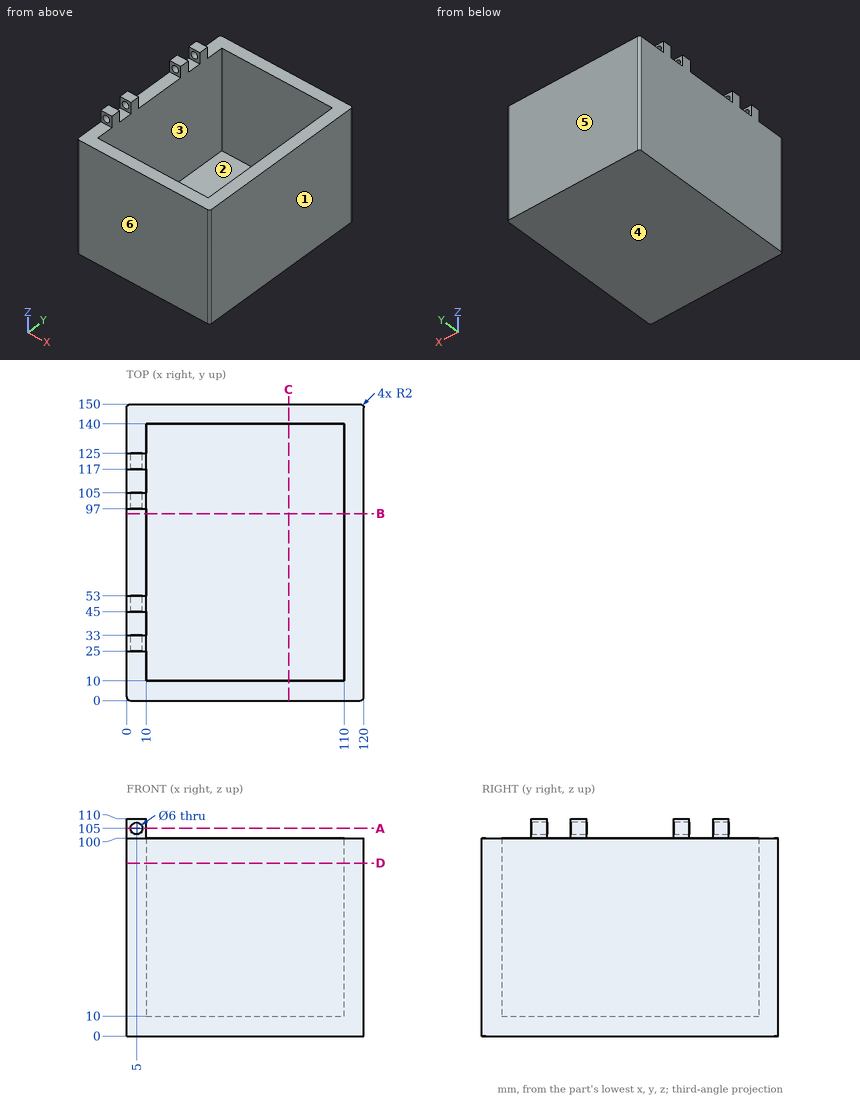
For this review, use the dimensioned drawing (mm, ordinates from the lowest corner) and the shaded views. A direction names the side the tool comes from. Round coordinates to 2 decimals unless told otherwise and drop trailing zeros. Order: outer loops, then holes, each group sorted by start corner. A loop starts at its lowest first (then second) coordinate and runs counter-clockwise, first axis right, second up. Notation, with made-up numbers: (67.5, 74.5) -> (98.5, 74.5) arc R29 cw to (98.5, 112.5) -> close; hole circle Ø9 at (32.5, 2.25). An arc over 180 degrees is marked (long way). Put each result on its own line as item: value.
Q1. Add section B-B on y = 94.5. Write out the cut boundary in (x, z), plus the area to 3 significant figures.
Check result:
outline: (0, 0) -> (120, 0) -> (120, 100) -> (110, 100) -> (110, 10) -> (10, 10) -> (10, 100) -> (0, 100) -> close
area: 3,000 mm2
Q2. For probe 1 along X at (y, z) = (119.5, 105); probe 2 along X at (y, z) = (31, 30.5); probe 3 along Y at (x, z) = (97, 33.5), list the stretches that pass through material, from the lowest coordinate up. Write a range as [from, to].
Check result:
probe 1: [0, 2], [8, 10]
probe 2: [0, 10], [110, 120]
probe 3: [0, 10], [140, 150]
Q3. Add section D-D on z = 87.5. Write out the cut boundary in (x, y).
Check result:
outline: (0, 2) arc R2 ccw to (2, 0) -> (118, 0) arc R2 ccw to (120, 2) -> (120, 148) arc R2 ccw to (118, 150) -> (2, 150) arc R2 ccw to (0, 148) -> close; hole (10, 10) -> (110, 10) -> (110, 140) -> (10, 140) -> close
Q4. Mouldability with a two-part tool opening along Y and no side actions: class the marked faces 3, 4, 5 and 6 as pulls with the +Y half, pulls with the -Y half, needs draft (parallel to the pull), parting line crosses it, or undercut.
Check result:
face 3: undercut
face 4: needs draft
face 5: pulls with the +Y half
face 6: pulls with the -Y half
Q5. Insertion check: pin 1 Ø10 at (x, y) = (30.5, 17) entering from +Z; pin 2 Ø5 at (x, z) = (6, 104.5) entering from -Y; pin 3 Ø5 at (x, z) = (5, 105) entering from -Y; pin 4 Ø8 at (x, y) = (13, 70.5) entering from +Z. Each pin has a flat end and moves straight along its axis. Give the tip position at first contact, or say it passes through.
Check result:
pin 1: z = 10
pin 2: y = 25
pin 3: through
pin 4: z = 100
Q6. Add section C-C on x = 82. Write out the cut boundary in (y, z).
Check result:
outline: (0, 0) -> (150, 0) -> (150, 100) -> (140, 100) -> (140, 10) -> (10, 10) -> (10, 100) -> (0, 100) -> close
Q7. Machinability: for the marked faces 1 and 2, which of the approach directions +Z, -Z, +X, -X, +Y, -Y give a long, thin tool a straight path to every point of the face, cutting with its end or side? Answer none if there is none.
Check result:
face 1: +Z, -Z, +X, +Y, -Y
face 2: +Z
Q8. Add section A-A on z = 105. State how many separate pieces and enclosed holes the cut face has, plus the area to 3 significant figures.
Check result:
separate pieces: 8
enclosed holes: 0
area: 128 mm2
